Verification items for the finished model (mm, model axes). A direction names the side the tool comes from. Coordinates: 2 decimals unless noted, no trailing zeros. Loops run counter-clockwise (first coordinate to the right, second up) from the corner with the lowest first, then second, coordinate; pieces in that order, holes last. Notation, with made-up numbers: (51, -18) -> (110, -18) arc R26 ccw to (110, -1) -> close; hole circle Ø9 at (7.25, 43.5). An arc over 180 degrees is marked (long way). Use CSV: the item, a comma, the result in double quotes. Start each with the question number.
```python
from build123d import *

# Parameters (mm, degrees)
SKETCH1_W                = 120
SKETCH1_H                = 120
MAIN_BODY_DEPTH          = 151
SKETCH11_W               = 114
SKETCH11_H               = 117
HOLLOW_DEPTH             = 148
SKETCH12_W               = 4
SKETCH12_H               = 148
BOSS_EXTRUDE1_DEPTH      = 10
SKETCH13_W               = 4
SKETCH13_H               = 148
BOSS_EXTRUDE2_DEPTH      = 10
LED_MOUNTING_HOLES_REACH = 175.208
SKETCH14_R               = 1.1
SKETCH15_R               = 1.5
LED_POSITION_DEPTH       = 1
BOLT_HOLE_1_REACH        = 203.993
SKETCH16_R               = 1.5
LPATTERN1_COUNT          = 2
LPATTERN1_PITCH          = 93.8
CUT_EXTRUDE5_DEPTH       = 2
SKETCH20_R               = 1.5
CUT_EXTRUDE6_DEPTH       = 10
SKETCH21_R               = 1.5
BOLT_HOLE1_DEPTH         = 10
NUT_HOLE1_DEPTH          = 2
NUT_HOLE3_DEPTH          = 2
SKETCH33_R               = 1.5
BOLT_HOLE3_DEPTH         = 12
NUT_HOLE4_DEPTH          = 2
SKETCH35_R               = 1.5
CUT_EXTRUDE16_DEPTH      = 12


with BuildPart() as part:
    # Sketch1 → Main-Body (new body)
    with BuildSketch(Plane(origin=(0, 0, 0), x_dir=(1, 0, 0), z_dir=(0, 1, 0))):
        Rectangle(SKETCH1_W, SKETCH1_H)
    extrude(amount=MAIN_BODY_DEPTH)

    # Sketch11 → Hollow (cut)
    with BuildSketch(Plane(origin=(0, 151, 0), x_dir=(1, 0, 0), z_dir=(0, 1, 0))):
        with Locations((0, -1.5)):
            Rectangle(SKETCH11_W, SKETCH11_H)
    extrude(amount=-HOLLOW_DEPTH, mode=Mode.SUBTRACT)

    # Sketch12 → Boss-Extrude1 (add)
    with BuildSketch(Plane.ZY.offset(-57)):
        with Locations((58, 77)):
            Rectangle(SKETCH12_W, SKETCH12_H)
    extrude(amount=BOSS_EXTRUDE1_DEPTH)

    # Sketch13 → Boss-Extrude2 (add)
    with BuildSketch(Plane(origin=(-57, 0, 0), x_dir=(0, 0, -1), z_dir=(1, 0, 0))):
        with Locations((-58, 77)):
            Rectangle(SKETCH13_W, SKETCH13_H)
    extrude(amount=BOSS_EXTRUDE2_DEPTH)

    # Sketch14 → LED-Mounting-Holes (cut, up to next)
    with BuildSketch(Plane(origin=(0, 0, 0), x_dir=(0, 0, 1), z_dir=(0, -1, 0)), mode=Mode.PRIVATE) as led_mounting_holes_sk1:
        with Locations(Location((-2.225, 9, 0), (0, 0, 180))):
            Circle(SKETCH14_R)
    led_mounting_holes_tool1 = extrude(led_mounting_holes_sk1.sketch, amount=-LED_MOUNTING_HOLES_REACH, mode=Mode.PRIVATE) & part.part
    # Sketch14 → LED-Mounting-Holes (cut, up to next)
    with BuildSketch(Plane(origin=(0, 0, 0), x_dir=(0, 0, 1), z_dir=(0, -1, 0)), mode=Mode.PRIVATE) as led_mounting_holes_sk2:
        with Locations(Location((5.275, 9, 0), (0, 0, 180))):
            Circle(SKETCH14_R)
    led_mounting_holes_tool2 = extrude(led_mounting_holes_sk2.sketch, amount=-LED_MOUNTING_HOLES_REACH, mode=Mode.PRIVATE) & part.part
    # Sketch14 → LED-Mounting-Holes (cut, up to next)
    with BuildSketch(Plane(origin=(0, 0, 0), x_dir=(0, 0, 1), z_dir=(0, -1, 0)), mode=Mode.PRIVATE) as led_mounting_holes_sk3:
        with Locations(Location((5.275, -9, 0), (0, 0, 180))):
            Circle(SKETCH14_R)
    led_mounting_holes_tool3 = extrude(led_mounting_holes_sk3.sketch, amount=-LED_MOUNTING_HOLES_REACH, mode=Mode.PRIVATE) & part.part
    # Sketch14 → LED-Mounting-Holes (cut, up to next)
    with BuildSketch(Plane(origin=(0, 0, 0), x_dir=(0, 0, 1), z_dir=(0, -1, 0)), mode=Mode.PRIVATE) as led_mounting_holes_sk4:
        with Locations(Location((-2.225, -9, 0), (0, 0, 180))):
            Circle(SKETCH14_R)
    led_mounting_holes_tool4 = extrude(led_mounting_holes_sk4.sketch, amount=-LED_MOUNTING_HOLES_REACH, mode=Mode.PRIVATE) & part.part
    add(led_mounting_holes_tool1.solids().sort_by_distance((-9, 0, -2.225))[0], mode=Mode.SUBTRACT)
    add(led_mounting_holes_tool2.solids().sort_by_distance((-9, 0, 5.275))[0], mode=Mode.SUBTRACT)
    add(led_mounting_holes_tool3.solids().sort_by_distance((9, 0, 5.275))[0], mode=Mode.SUBTRACT)
    add(led_mounting_holes_tool4.solids().sort_by_distance((9, 0, -2.225))[0], mode=Mode.SUBTRACT)

    # Sketch15 → LED-Position (cut)
    with BuildSketch(Plane(origin=(0, 3, 0), x_dir=(1, 0, 0), z_dir=(0, 1, 0))):
        with Locations(Location((0, -0.05, 0), (0, 0, 270))):
            Circle(SKETCH15_R)
    extrude(amount=-LED_POSITION_DEPTH, mode=Mode.SUBTRACT)

    # Sketch16 → Bolt-Hole-1 (cut, up to next)
    with BuildSketch(Plane(origin=(0, 0, -60), x_dir=(-1, 0, 0), z_dir=(0, 0, -1)), mode=Mode.PRIVATE) as bolt_hole_1_sk1:
        with Locations((-46.9, 143)):
            Circle(SKETCH16_R)
    bolt_hole_1_tool1 = extrude(bolt_hole_1_sk1.sketch, amount=-BOLT_HOLE_1_REACH, mode=Mode.PRIVATE) & part.part
    bolt_hole_1 = bolt_hole_1_tool1.solids().sort_by_distance((46.9, 143, -60))[0]
    add(bolt_hole_1, mode=Mode.SUBTRACT)

    # LPattern1: Bolt-Hole-1 ×2
    with Locations(*[(-i * LPATTERN1_PITCH, 0, 0) for i in range(1, LPATTERN1_COUNT)]):
        add(bolt_hole_1, mode=Mode.SUBTRACT)

    # Sketch18 → Cut-Extrude5 (cut)
    with BuildSketch(Plane(origin=(0, 0, 56), x_dir=(-1, 0, 0), z_dir=(0, 0, -1))):
        Polygon((55.2, 136), (53.6, 138.771281292), (50.4, 138.771281292), (48.8, 136), (50.4, 133.228718708), (53.6, 133.228718708), align=None)
    extrude(amount=-CUT_EXTRUDE5_DEPTH, mode=Mode.SUBTRACT)

    # Sketch20 → Cut-Extrude6 (cut)
    with BuildSketch(Plane(origin=(0, 0, 58), x_dir=(-1, 0, 0), z_dir=(0, 0, -1))):
        with Locations((52, 136)):
            Circle(SKETCH20_R)
    extrude(amount=-CUT_EXTRUDE6_DEPTH, mode=Mode.SUBTRACT)

    # Sketch21 → Bolt-Hole1 (cut)
    with BuildSketch(Plane(origin=(0, 0, 56), x_dir=(-1, 0, 0), z_dir=(0, 0, -1))):
        with Locations(Location((52, 36, 0), (0, 0, 90))):
            Circle(SKETCH21_R)
    extrude(amount=-BOLT_HOLE1_DEPTH, mode=Mode.SUBTRACT)

    # Sketch29 → Nut-hole1 (cut)
    with BuildSketch(Plane(origin=(0, 0, 56), x_dir=(-1, 0, 0), z_dir=(0, 0, -1))):
        Polygon((55.2, 36), (53.6, 38.771281292), (50.4, 38.771281292), (48.8, 36), (50.4, 33.228718708), (53.6, 33.228718708), align=None)
    extrude(amount=-NUT_HOLE1_DEPTH, mode=Mode.SUBTRACT)

    # Sketch32 → Nut-Hole3 (cut)
    with BuildSketch(Plane(origin=(0, 0, 56), x_dir=(-1, 0, 0), z_dir=(0, 0, -1))):
        Polygon((-48.8, 136), (-50.4, 138.771281292), (-53.6, 138.771281292), (-55.2, 136), (-53.6, 133.228718708), (-50.4, 133.228718708), align=None)
    extrude(amount=-NUT_HOLE3_DEPTH, mode=Mode.SUBTRACT)

    # Sketch33 → Bolt-Hole3 (cut)
    with BuildSketch(Plane(origin=(0, 0, 56), x_dir=(-1, 0, 0), z_dir=(0, 0, -1))):
        with Locations((-52, 136)):
            Circle(SKETCH33_R)
    extrude(amount=-BOLT_HOLE3_DEPTH, mode=Mode.SUBTRACT)

    # Sketch34 → Nut-hole4 (cut)
    with BuildSketch(Plane(origin=(0, 0, 56), x_dir=(-1, 0, 0), z_dir=(0, 0, -1))):
        Polygon((-48.8, 36), (-50.4, 38.771281292), (-53.6, 38.771281292), (-55.2, 36), (-53.6, 33.228718708), (-50.4, 33.228718708), align=None)
    extrude(amount=-NUT_HOLE4_DEPTH, mode=Mode.SUBTRACT)

    # Sketch35 → Cut-Extrude16 (cut)
    with BuildSketch(Plane(origin=(0, 0, 56), x_dir=(-1, 0, 0), z_dir=(0, 0, -1))):
        with Locations((-52, 36)):
            Circle(SKETCH35_R)
    extrude(amount=-CUT_EXTRUDE16_DEPTH, mode=Mode.SUBTRACT)


solid = part.part
```
1. Cross-section at B-B, the plane z = -33. Record the boundary of the cut face in (x, y), plus the area to 3 significant figures.
2. Release check for a two-part mould opening along Y. For faces 1 (the flat face through (47, 78, 58)), 2 (the flat face through (50.6, 137.3, 58)), 3 (the flat face through (-1, 0, -1)) record: released by +Y, released by -Y, zero draft, split by the parting line, or undercut.
3. Depth check by flat-ended pin: pin 1 (1 mm diameter, centred on x = -29.5, z = 30, fed in from +Y); pin 2 (2.5 mm diameter, centred on x = -9, z = 5.275, fed in from -Y); pin 3 (2.5 mm diameter, centred on x = 0, z = 0.05, fed in from +Y); pin 4 (2.5 mm diameter, centred on x = -52, y = 136, fed in from +Z). Enter the tip coordinate at first touch or a pass-through.
4. Set-up check for faces 4 (the flat face through (-53.4, 37.3, 58)), 5 (the flat face through (-47, 78, 58)), 6 (the flat face through (-57, 78, 0)): record each of +Z, -Z, +X, -X, +Y, -Y from which the full face is reachable in a straight line by a thin tool's end or side.
5. Cross-section at C-C, the plane y = 19.5. Record the boundary of the cut face in (x, z).
6. Scan lines: line 1 (Y direction, x = 52, z = 58.8); line 2 (X direction, y = 136, z = 58.75); line 3 (X direction, y = 113.5, z = -38.5). Record each from-to range of solid material in increasing order.
7. Cross-section at A-A, the plane x = 37. Record the boundary of the cut face in (y, z).
Solution:
1,outline,"(-60, 0) -> (60, 0) -> (60, 151) -> (57, 151) -> (57, 3) -> (-57, 3) -> (-57, 151) -> (-60, 151) -> close"
1,area,"1,250 mm2"
2,face 1,"zero draft"
2,face 2,"undercut"
2,face 3,"released by -Y"
3,pin 1,"stops at y = 3"
3,pin 2,"stops at y = 0"
3,pin 3,"stops at y = 2"
3,pin 4,"stops at z = -57"
4,face 4,"none"
4,face 5,"+Z, +Y"
4,face 6,"+Y"
5,outline,"(-60, -60) -> (60, -60) -> (60, 60) -> (47, 60) -> (47, 56) -> (57, 56) -> (57, -57) -> (-57, -57) -> (-57, 56) -> (-47, 56) -> (-47, 60) -> (-60, 60) -> close"
6,line 1,"y = 0 to 34.5, 37.5 to 134.5, 137.5 to 151"
6,line 2,"x = -60 to -53.5, -50.5 to -47, 47 to 50.5, 53.5 to 60"
6,line 3,"x = -60 to -57, 57 to 60"
7,outline,"(0, -60) -> (151, -60) -> (151, -57) -> (3, -57) -> (3, 60) -> (0, 60) -> close"
